from build123d import *

# Parameters (mm, degrees)
SKETCH1_W           = 47.5
SKETCH1_H           = 110
SKETCH1_R           = 2
SKETCH1_W_2         = 10
SKETCH1_H_2         = 10
BOSS_EXTRUDE1_DEPTH = 4
SKETCH2_R           = 12.5
SKETCH2_R_2         = 7.5
BOSS_EXTRUDE2_DEPTH = 30
SKETCH4_R           = 12.5
SKETCH4_R_2         = 7.5
BOSS_EXTRUDE3_DEPTH = 60


with BuildPart() as part:
    # Sketch1 → Boss-Extrude1 (new body)
    with BuildSketch(Plane(origin=(0, 0, 0), x_dir=(1, 0, 0), z_dir=(0, 1, 0))):
        with Locations((-12.897727273, -28.125)):
            Rectangle(SKETCH1_W, SKETCH1_H)
        with Locations(Location((0.852272727, 17.315, 0), (0, 0, 270))):
            Circle(SKETCH1_R, mode=Mode.SUBTRACT)
        with Locations(Location((-29.147727273, -8.845, 0), (0, 0, 270))):
            Circle(SKETCH1_R, mode=Mode.SUBTRACT)
        with Locations(Location((0.852272727, -45.685, 0), (0, 0, 270))):
            Circle(SKETCH1_R, mode=Mode.SUBTRACT)
        with Locations(Location((0.852272727, -74.045, 0), (0, 0, 270))):
            Circle(SKETCH1_R, mode=Mode.SUBTRACT)
        with Locations(Location((-29.147727273, -74.045, 0), (0, 0, 270))):
            Circle(SKETCH1_R, mode=Mode.SUBTRACT)
        with Locations((-14.147727273, 1.875)):
            Rectangle(SKETCH1_W_2, SKETCH1_H_2, mode=Mode.SUBTRACT)
        with Locations((-14.147727273, -48.125)):
            Rectangle(SKETCH1_W_2, SKETCH1_H_2, mode=Mode.SUBTRACT)
    extrude(amount=-BOSS_EXTRUDE1_DEPTH)

    # Sketch2 → Boss-Extrude2 (add)
    with BuildSketch(Plane(origin=(0, 0, 0), x_dir=(1, 0, 0), z_dir=(0, 1, 0))):
        with Locations(Location((-14.147727273, -48.125, 0), (0, 0, 270))):
            Circle(SKETCH2_R)
        with Locations(Location((-14.147727273, -48.125, 0), (0, 0, 270))):
            Circle(SKETCH2_R_2, mode=Mode.SUBTRACT)
    extrude(amount=BOSS_EXTRUDE2_DEPTH)

    # Sketch4 → Boss-Extrude3 (add)
    with BuildSketch(Plane(origin=(0, 0, 0), x_dir=(1, 0, 0), z_dir=(0, 1, 0))):
        with Locations(Location((-14.147727273, 1.875, 0), (0, 0, 270))):
            Circle(SKETCH4_R)
        with Locations(Location((-14.147727273, 1.875, 0), (0, 0, 270))):
            Circle(SKETCH4_R_2, mode=Mode.SUBTRACT)
    extrude(amount=BOSS_EXTRUDE3_DEPTH)


solid = part.part
Verification items for the finished model (mm, model axes). A direction names the side the tool comes from. Give positions to 0.01 mm unless a question says otherwise; leave off trailing zeros. Loops run counter-clockwise (first coordinate to the right, second up) from the corner with the lowest first, then second, coordinate; pieces in that order, holes last.
1) Sectioned sample at A-A, the plane x = -11. Enter the section's corners in (y, z) (3 decimals).
2) Depth check by flat-ended pin: pin 1 Ø4 at (x, z) = (0.5, -15.5) entering from +Y; pin 2 Ø3 at (x, z) = (-29.15, 8.85) entering from -Y; pin 3 Ø3 at (x, y) = (-13, 8.5) entering from -Z (3 decimals); pin 4 Ø8 at (x, y) = (-19, 15) entering from +Z. Enter the tip coordinate at first touch or a pass-through.
3) Set-up check for faces 1 (the flat face through (-14, -2, 43.125)), 2 (the flat face through (-20, 30, 54)), 3 (the cylindrical face through (-20.8, 29.58, 1.59)): record each of +Z, -Z, +X, -X, +Y, -Y from which the full face is reachable in a straight line by a thin tool's end or side.
4) Sectioned sample at C-C, the plane z = 59. Enter the section's corners in (x, y).
5) Draft check along Z on faces 4 (the flat face through (-14, -2, -6.875)), 5 (the cylindrical face through (0.94, -1.972, -19.313)), 6 (the flat face through (10.852, -2, 29)). Enter one of: pulls with the +Z half, pulls with the -Z half, needs draft (parallel to the pull), parting line crosses it, or undercut.
6) Sectioned sample at B-B, the plane y = 2.5. Enter the section's corners in (x, z) (3 decimals), then the cut area to 3 significant figures.
7) Sectioned sample at D-D, the plane x = -3. Enter the section's corners in (y, z) (3 decimals), then the cut area to 3 significant figures.
8) Thickness scan on line 1 along Z through (x, y) = (-15, 20); line 2 along Z through (x, y) = (-19, 24); line 3 along Y through (x, z) = (-25, 26). Record the ranges inside material, lowest first.
Answers:
1. outline: (-4, -26.875) - (0, -26.875) - (0, -13.972) - (60, -13.972) - (60, -8.682) - (0, -8.682) - (0, -6.875) - (-4, -6.875) - close; (-4, 3.125) - (0, 3.125) - (0, 4.932) - (60, 4.932) - (60, 10.222) - (0, 10.222) - (0, 36.028) - (30, 36.028) - (30, 41.318) - (0, 41.318) - (0, 43.125) - (-4, 43.125) - close; (-4, 53.125) - (0, 53.125) - (0, 54.932) - (30, 54.932) - (30, 60.222) - (0, 60.222) - (0, 83.125) - (-4, 83.125) - close
2. pin 1: stops at y = 0
2. pin 2: passes through
2. pin 3: stops at z = -14.375
2. pin 4: stops at z = 60.6
3. face 1: +Y, -Y
3. face 2: +Z, +X, -X, +Y
3. face 3: +Y
4. outline: (-36.65, -4) - (10.85, -4) - (10.85, 0) - (-7.98, 0) - (-7.98, 30) - (-20.31, 30) - (-20.31, 0) - (-36.65, 0) - close
5. face 4: undercut
5. face 5: undercut
5. face 6: needs draft
6. outline: circle Ø25 at (-14.148, -1.875); circle Ø25 at (-14.148, 48.125); hole circle Ø15 at (-14.148, -1.875); hole circle Ø15 at (-14.148, 48.125)
6. area: 628 mm2
7. outline: (-4, -26.875) - (0, -26.875) - (0, -7.53) - (60, -7.53) - (60, 3.78) - (0, 3.78) - (0, 42.47) - (30, 42.47) - (30, 53.78) - (0, 53.78) - (0, 83.125) - (-4, 83.125) - close
7. area: 1,460 mm2
8. line 1: z = -14.35 to -9.33, 5.58 to 10.6, 35.65 to 40.67, 55.58 to 60.6
8. line 2: z = -13.39 to -7.59, 3.84 to 9.64, 36.61 to 42.41, 53.84 to 59.64
8. line 3: y = -4 to 0
